The listing builds one solid part. Answer for the finished solid, in the listing's coordinates (mm). A direction names the side the tool comes from. Coordinates: 2 decimals unless noted, no trailing zeros. Order: outer loops, then holes, each group sorted by start corner. A loop starts at its lowest first (then second) coordinate and runs counter-clockwise, first axis right, second up. Notation, with made-up numbers: (-19, 41) -> (39, 41) arc R34 ccw to (39, 76) -> close; hole circle Ø7 at (46, 23.25). An arc over 180 degrees is marked (long way). Write item = value, one per line.
Autodesk Inventor part; units mm, degrees
ref_plane "Work Plane2" through (0, 0, 208.9658) normal (0, 0, 1) x (1, 0, 0)
ref_plane "YZ Plane" through (0, 0, 0) normal (1, 0, 0) x (0, 1, 0)
ref_plane "XZ Plane" through (0, 0, 0) normal (0, 1, 0) x (-1, 0, 0)
ref_plane "Work Plane1" through (0, 0, 0) normal (0, 0, 1) x (1, 0, 0)
sketch "Sketch1" plane through (0, 0, 0) normal (0, 0, 1) x (1, 0, 0)
  arc A0 (-113.2188, 0) -> (-109.7581, 3.4607) centre (-113.2188, 3.4607) ccw
  line L0 (-109.7581, 17.1767) -> (-109.7581, 3.4607)
  arc A1 (-109.7581, 17.1767) -> (-114.8063, 22.225) centre (-114.8063, 17.1767) ccw
  line L1 (-115.8223, 22.225) -> (-114.8063, 22.225)
  arc A2 (-115.8223, 22.225) -> (-119.2831, 18.7642) centre (-115.8223, 18.7642) ccw
  line L2 (-119.2831, 16.4211) -> (-119.2831, 18.7642)
  arc A3 (-119.2831, 16.4211) -> (-116.6161, 16.4211) centre (-117.9496, 16.4211) ccw
  line L3 (-116.6161, 18.7642) -> (-116.6161, 16.4211)
  arc A4 (-115.8223, 19.558) -> (-116.6161, 18.7642) centre (-115.8223, 18.7642) ccw
  line L4 (-114.8063, 19.558) -> (-115.8223, 19.558)
  arc A5 (-112.4251, 17.1767) -> (-114.8063, 19.558) centre (-114.8063, 17.1767) ccw
  line L5 (-112.4251, 3.4607) -> (-112.4251, 17.1767)
  arc A6 (-113.2188, 2.667) -> (-112.4251, 3.4607) centre (-113.2188, 3.4607) ccw
  line L6 (-147.5723, 2.667) -> (-113.2188, 2.667)
  arc A7 (-148.3661, 3.4607) -> (-147.5723, 2.667) centre (-147.5723, 3.4607) ccw
  line L7 (-148.3661, 17.1767) -> (-148.3661, 3.4607)
  arc A8 (-145.9848, 19.558) -> (-148.3661, 17.1767) centre (-145.9848, 17.1767) ccw
  line L8 (-144.9688, 19.558) -> (-145.9848, 19.558)
  arc A9 (-144.1751, 18.7642) -> (-144.9688, 19.558) centre (-144.9688, 18.7642) ccw
  line L9 (-144.1751, 16.4211) -> (-144.1751, 18.7642)
  arc A10 (-144.1751, 16.4211) -> (-141.5081, 16.4211) centre (-142.8416, 16.4211) ccw
  line L10 (-141.5081, 18.7642) -> (-141.5081, 16.4211)
  arc A11 (-141.5081, 18.7642) -> (-144.9688, 22.225) centre (-144.9688, 18.7642) ccw
  line L11 (-145.9848, 22.225) -> (-144.9688, 22.225)
  arc A12 (-145.9848, 22.225) -> (-151.0331, 17.1767) centre (-145.9848, 17.1767) ccw
  line L12 (-151.0331, 3.4607) -> (-151.0331, 17.1767)
  arc A13 (-151.0331, 3.4607) -> (-147.5723, 0) centre (-147.5723, 3.4607) ccw
  line L13 (-113.2188, 0) -> (-147.5723, 0)
  point P0 (0, 0)
extrude "Extrusion1" add sketch "Sketch1" along normal blind 417.9316
ref_plane "Work Plane2" through (0, 0, 208.9658) normal (0, 0, 1) x (1, 0, 0)
sketch "Sketch2" plane through (-147.5723, 0, 0) normal (0, -1, 0) x (1, 0, 0)
  line L0 (17.1768, 26.4541) -> (17.1768, 40.7289) construction
  line L1 (6.0642, 0) -> (6.0642, 417.9316)
  line L2 (10.0267, 26.4541) -> (10.0267, 40.7289)
  line L3 (24.3269, 40.7289) -> (24.3269, 26.4541)
  arc A0 (10.0267, 26.4541) -> (24.3269, 26.4541) centre (17.1768, 26.4541) ccw
  arc A1 (24.3269, 40.7289) -> (10.0267, 40.7289) centre (17.1768, 40.7289) ccw
  line L4 (0, 0) -> (34.3535, 0) construction
  line L5 (17.1768, 0) -> (17.1767, 417.9316) construction
  line L6 (34.3535, 417.9316) -> (0, 417.9316) construction
  line L7 (10.0267, 77.2541) -> (10.0267, 91.5289)
  line L8 (24.3269, 91.5289) -> (24.3269, 77.2541)
  arc A2 (10.0267, 77.2541) -> (24.3269, 77.2541) centre (17.1768, 77.2541) ccw
  arc A3 (24.3269, 91.5289) -> (10.0267, 91.5289) centre (17.1768, 91.5289) ccw
  line L9 (17.1768, 50.8) -> (17.1767, 468.7316) construction
  line L10 (10.0266, 128.0541) -> (10.0266, 142.3289)
  line L11 (24.3268, 142.3289) -> (24.3268, 128.0541)
  arc A4 (10.0266, 128.0541) -> (24.3268, 128.0541) centre (17.1767, 128.0541) ccw
  arc A5 (24.3268, 142.3289) -> (10.0266, 142.3289) centre (17.1767, 142.3289) ccw
  line L12 (17.1768, 101.6) -> (17.1767, 519.5316) construction
  line L13 (10.0266, 178.8541) -> (10.0266, 193.1289)
  line L14 (24.3268, 193.1289) -> (24.3268, 178.8541)
  arc A6 (10.0266, 178.8541) -> (24.3268, 178.8541) centre (17.1767, 178.8541) ccw
  arc A7 (24.3268, 193.1289) -> (10.0266, 193.1289) centre (17.1767, 193.1289) ccw
  line L15 (17.1767, 152.4) -> (17.1767, 570.3316) construction
  line L16 (10.0266, 229.6541) -> (10.0266, 243.9289)
  line L17 (24.3268, 243.9289) -> (24.3268, 229.6541)
  arc A8 (10.0266, 229.6541) -> (24.3268, 229.6541) centre (17.1767, 229.6541) ccw
  arc A9 (24.3268, 243.9289) -> (10.0266, 243.9289) centre (17.1767, 243.9289) ccw
  line L18 (17.1767, 203.2) -> (17.1767, 621.1316) construction
  line L19 (10.0266, 280.4541) -> (10.0266, 294.7289)
  line L20 (24.3268, 294.7289) -> (24.3268, 280.4541)
  arc A10 (10.0266, 280.4541) -> (24.3268, 280.4541) centre (17.1767, 280.4541) ccw
  arc A11 (24.3268, 294.7289) -> (10.0266, 294.7289) centre (17.1767, 294.7289) ccw
  line L21 (17.1767, 254) -> (17.1767, 671.9316) construction
  line L22 (10.0266, 331.2541) -> (10.0266, 345.5289)
  line L23 (24.3268, 345.5289) -> (24.3268, 331.2541)
  arc A12 (10.0266, 331.2541) -> (24.3268, 331.2541) centre (17.1767, 331.2541) ccw
  arc A13 (24.3268, 345.5289) -> (10.0266, 345.5289) centre (17.1767, 345.5289) ccw
  line L24 (17.1767, 304.8) -> (17.1767, 722.7316) construction
  line L25 (10.0266, 382.0541) -> (10.0266, 396.3289)
  line L26 (24.3268, 396.3289) -> (24.3268, 382.0541)
  arc A14 (10.0266, 382.0541) -> (24.3268, 382.0541) centre (17.1767, 382.0541) ccw
  arc A15 (24.3268, 396.3289) -> (10.0266, 396.3289) centre (17.1767, 396.3289) ccw
  line L27 (17.1767, 355.6) -> (17.1767, 773.5316) construction
  point P0 (147.5723, 0)
  point P1 (17.1768, 33.5915)
  point P2 (17.1768, 84.3915)
  point P3 (17.1768, 135.1915)
  point P4 (17.1767, 185.9915)
  point P5 (17.1767, 236.7915)
  point P6 (17.1767, 287.5915)
  point P7 (17.1767, 338.3915)
  point P8 (17.1767, 389.1915)
  dimension "d2" = 14.3002
  dimension "d3" = 14.2748
  dimension "d4" = 26.4541
  dimension "d7" = 50.8
extrude "Extrusion2" cut sketch "Sketch2" against normal blind 25.4
properties part number "Horizontal-Unistrut-Tower-Connector-15"
Q1. Section C-C, the plane z = 63 is taken. Give the vertices of the cut face in (x, y) (1 decimal).
The answers:
outline = (-151, 3.5) arc R3.5 ccw to (-147.6, 0) -> (-113.2, 0) arc R3.5 ccw to (-109.8, 3.5) -> (-109.8, 17.2) arc R5 ccw to (-114.8, 22.2) -> (-115.8, 22.2) arc R3.5 ccw to (-119.3, 18.8) -> (-119.3, 16.4) arc R1.3 ccw to (-116.6, 16.4) -> (-116.6, 18.8) arc R0.8 cw to (-115.8, 19.6) -> (-114.8, 19.6) arc R2.4 cw to (-112.4, 17.2) -> (-112.4, 3.5) arc R0.8 cw to (-113.2, 2.7) -> (-147.6, 2.7) arc R0.8 cw to (-148.4, 3.5) -> (-148.4, 17.2) arc R2.4 cw to (-146, 19.6) -> (-145, 19.6) arc R0.8 cw to (-144.2, 18.8) -> (-144.2, 16.4) arc R1.3 ccw to (-141.5, 16.4) -> (-141.5, 18.8) arc R3.5 ccw to (-145, 22.2) -> (-146, 22.2) arc R5 ccw to (-151, 17.2) -> close
Q2. Each of these flat-tipped pins is pushed along its axis until it touches: pin 1 Ø2 at (y, z) = (1, 235.5) entering from -X; pin 2 Ø2 at (y, z) = (0.5, 341) entering from -X; pin 3 Ø1 at (x, z) = (-114, 243.5) entering from +Y; pin 4 Ø1.5 at (x, z) = (-127, 145.5) entering from -Y. Where does it stop, or does it pass through?
The answers:
pin_1 = -150.71
pin_2 = -150.42
pin_3 = 22.22
pin_4 = through
Q3. The mould has two halves that part along Y. Classify faces 1 (the face through (-148.366, 10, 206)), 2 (the face through (-130, 2, 417.932)), 3 (the face through (-130, 0, 206)): released by +Y, released by -Y, zero draft, split by the parting line, or undercut.
The answers:
face_1 = undercut
face_2 = zero draft
face_3 = released by -Y
Q4. A tool of negligible diameter and unlimited length cuts with its end or side. For faces 4 (the face through (-112.425, 10, 206)), 5 (the face through (-151.033, 10, 206)), 6 (the face through (-130.238, 1.315, 301.877)), from which of +Z, -Z, +X, -X, +Y, -Y can it reach the whole face along a straight path? Write none if from no direction.
The answers:
face_4 = +Z, -Z
face_5 = +Z, -Z, -X, +Y, -Y
face_6 = +Y, -Y
Q5. Section B-B, the plane y = 8.5 is taken. Give the vertices of the cut face in (x, z).
The answers:
outline = (-151.03, 0) -> (-148.37, 0) -> (-148.37, 417.93) -> (-151.03, 417.93) -> close; (-112.43, 0) -> (-109.76, 0) -> (-109.76, 417.93) -> (-112.43, 417.93) -> close
Q6. Find the intervals of material crossed by line 1 along X through (y, z) = (17, 321); line 2 along X through (y, z) = (6.75, 312.5); line 3 along X through (y, z) = (17.75, 207.5), in increasing order.
The answers:
line_1 = -151.03 to -148.37, -144.18 to -141.51, -119.28 to -116.62, -112.43 to -109.76
line_2 = -151.03 to -148.37, -112.43 to -109.76
line_3 = -151 to -148.3, -144.18 to -141.51, -119.28 to -116.62, -112.5 to -109.79
